Autodesk Inventor part; units mm, degrees
ref_plane "YZ Plane" through (0, 0, 0) normal (1, 0, 0) x (0, 1, 0)
ref_plane "XZ Plane" through (0, 0, 0) normal (0, 1, 0) x (-1, 0, 0)
ref_plane "XY Plane" through (0, 0, 0) normal (0, 0, 1) x (1, 0, 0)
sketch "Skizze1" plane through (0, 0, 0) normal (1, 0, 0) x (0, 1, 0)
  line L0 (0, 0) -> (16, 0)
  line L1 (16, 0) -> (16, -16)
  line L2 (16, -16) -> (0, -16)
  line L3 (0, -16) -> (0, 0)
  dimension "d0" = 16
  dimension "d1" = 16
extrude "Extrusion1" add sketch "Skizze1" along normal blind 16
sketch "Skizze2" plane through (0, 16, 0) normal (0, 1, 0) x (1, 0, 0)
  line L0 (5, 8) -> (0, 8)
  line L1 (0, 16) -> (0, 0)
  dimension "d4" = 5
hole "Bohrung1" at (5, 16, -8) direction (0, -1, 0) diameter 4.3 end through all countersink diameter 11 countersink angle 90
sketch "Skizze3" plane through (0, 0, 0) normal (0, 0, 1) x (1, 0, 0)
  line L0 (0, 16) -> (0, 0)
  line L1 (0, 8) -> (8, 8)
  dimension "d12" = 8
hole "Bohrung2" at (8, 8, 0) direction (0, 0, -1) diameter 2.459 end through all
sketch "Skizze4" plane through (16, 0, 0) normal (1, 0, 0) x (0, 0, -1)
  line L0 (10.15, 0) -> (5.85, 0)
  line L1 (8, 0) -> (8, 8)
  point P0 (0, 0)
  dimension "d20" = 8
hole "Bohrung3" at (16, 8, -8) direction (-1, 0, 0) diameter 2.459 end through all
properties part number "Frameblock" material "PC/ABS-Kunststoff, 3DDruck, PLA"
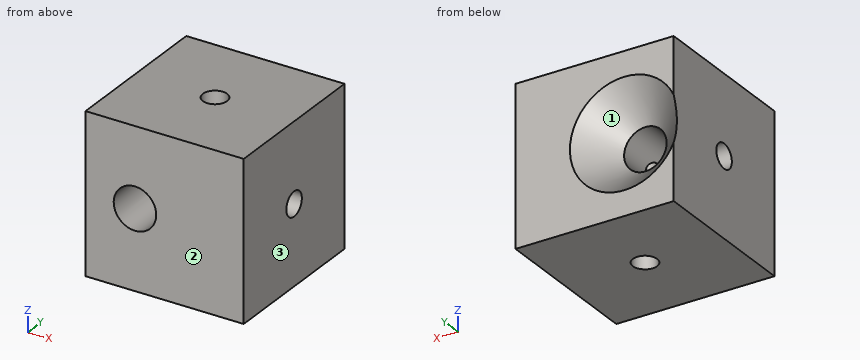
Can you work these out from the model? Positions are in its coordinate system, mm. Face numbers are marked on the shaded views. Coordinates: 2 decimals unless noted, no trailing zeros. Order: outer loops, then holes, each group sorted by start corner. A loop starts at its lowest first (then second) coordinate and runs counter-clockwise, first axis right, second up. Notation, with made-up numbers: (-5, -4) - (19, -4) arc R12 ccw to (19, 1) - close; hole circle Ø11 at (7, 56.5). An arc over 180 degrees is marked (long way). Answer in a Markdown table with one row per item.
1. Suppose I cut it at B-B (x = 13.75). Please give me the cut outline in (y, z), and give its area (3 significant figures).
Reply:
| item | result |
|---|---|
| outline | (0, -16) - (16, -16) - (16, 0) - (0, 0) - close; hole circle Ø2.46 at (8, -8) |
| area | 251 mm^2 |
2. If I drill on line 1 along Z through (x, y) = (13.75, 8); line 2 along X through (y, z) = (8, -13.5), over which ranges is the centre line in solid material (lowest first)?
Reply:
| item | result |
|---|---|
| line 1 | z = -16 to -9.23, -6.77 to 0 |
| line 2 | x = 0 to 6.77, 9.23 to 16 |
3. Suppose I cut it at D-D (x = 5). Please give me the cut outline in (y, z).
Reply:
| item | result |
|---|---|
| outline | (0, -16) - (16, -16) - (16, -13.5) - (12.65, -10.15) - (0, -10.15) - close; (0, -5.85) - (12.65, -5.85) - (16, -2.5) - (16, 0) - (0, 0) - close |
4. If we mould it in two halves opening along X, with no side actions, what happens to the marked faces 1, 2 and 3? For each: pulls with the +X half, pulls with the -X half, needs draft (parallel to the pull), parting line crosses it, or undercut.
Reply:
| item | result |
|---|---|
| face 1 | undercut |
| face 2 | needs draft |
| face 3 | pulls with the +X half |
5. Suppose I cut it at A-A (y = 8). Give the number of separate pieces and of enclosed holes in the cut face, and give its area (3 significant figures).
Reply:
| item | result |
|---|---|
| separate pieces | 4 |
| enclosed holes | 0 |
| area | 179 mm^2 |
6. Suppose I cut it at C-C (z = -15). Please give me the cut outline in (x, y).
Reply:
| item | result |
|---|---|
| outline | (0, 0) - (16, 0) - (16, 16) - (0, 16) - close; hole circle Ø2.46 at (8, 8) |
